The model under review builds one solid part; all positions refer to its coordinate system, in mm. A direction names the side the tool comes from. Coordinates: 2 decimals unless noted, no trailing zeros. Write each loop counter-clockwise with the first axis right and the second up, starting at its lowest first coordinate (ties: lowest second). Pieces come first, ordered by that corner, then holes. Notation, with made-up numbers: (-6, 36.5) - (38, 36.5) arc R9 cw to (38, 42.5) - close; hole circle Ø3 at (2.25, -27). An arc over 180 degrees is marked (long way). Put each result on its own line as item: value. Start each with the question number.
Item 1: Machinability: for faces 1 (the face through (1.115, 41.855, 5.022)), 2 (the face through (0.07, 13, 14.15)), 3 (the face through (-12.932, 6.409, 5.362)), which of the approach directions +Z, -Z, +X, -X, +Y, -Y give a long, thin tool a straight path to every point of the face, cutting with its end or side? Answer none if there is none.
Item 2: Consider section D-D on y = 40.5. Give the boundary of the cut face in (x, z), then the cut area to 3 significant figures.
Item 3: Consider section A-A on y = 5. State how many separate pieces and enclosed holes the cut face has, then the cut area to 3 significant figures.
Item 4: To check wall thickness, follow L1, parallel to Y at x = -11, z = -11; L2, parallel to Y at x = -10, z = -11; L3, parallel to X at y = 23.5, z = 1. State the ranges of each line that lie inside material, in increasing order. Write a range as [from, to].
Item 5: Consider section B-B on y = 23. Give the boundary of the cut face in (x, z).
Item 6: Mouldability with a two-part tool opening along X and no side actions: class faces 4 (the face through (4.119, 19.126, 18.548)), 5 (the face through (-6, 0, -13)), 6 (the face through (3.47, 19.78, 15.62)) as pulls with the +X half, pulls with the -X half, needs draft (parallel to the pull), parting line crosses it, or undercut.
Item 7: For pin 1 (10 mm diameter, centred on x = -6, z = -6.5, fed in from -Y); pin 2 (2 mm diameter, centred on y = 40.5, z = 8.5, fed in from -X); pin 3 (3 mm diameter, centred on x = 3, z = 2, fed in from -Y); pin 4 (1 mm diameter, centred on x = -10, y = 14.5, fed in from -Z), all flat-tipped, find the tip position at first contact; note any pin that passes through.
```python
from build123d import *

# Parameters (mm, degrees)
SKETCH3_R          = 1.5
CUT_EXTRUDE1_DEPTH = 55.138710735
CIRPATTERN1_COUNT  = 8


with BuildPart() as part:
    # Sketch2 → Revolve1 (revolve)
    with BuildSketch(Plane.XY, mode=Mode.PRIVATE) as revolve1_sk:
        Polygon((17, 0), (17, 10), (19, 10), (19, 28), (0, 47), (0, 42.757359313), (16, 26.757359313), (16, 13), (14, 13), (14, 0), align=None)
    revolve(revolve1_sk.sketch.rotate(Axis((0, 26.112729166, 0), (0, -1, 0)), 180), axis=Axis((0, 26.112729166, 0), (0, -1, 0)))

    # Sketch3 → Cut-Extrude1 (cut, through all)
    with BuildSketch(Plane.XY):
        with Locations((0, 5)):
            Circle(SKETCH3_R)
    cut_extrude1 = extrude(amount=-CUT_EXTRUDE1_DEPTH, mode=Mode.SUBTRACT)

    # CirPattern1: Cut-Extrude1 ×8 about axis
    cirpattern1_axis = Axis((0, 26.112729166, 0), (0, 1, 0))
    for i in range(1, CIRPATTERN1_COUNT):
        add(cut_extrude1.rotate(cirpattern1_axis, i * 360 / CIRPATTERN1_COUNT), mode=Mode.SUBTRACT)


solid = part.part
```
Report:
1. face 1: +Y
1. face 2: none
1. face 3: -Y
2. outline: circle Ø13 at (0, 0); hole circle Ø4.51 at (0, 0)
2. area: 117 mm²
3. separate pieces: 8
3. enclosed holes: 0
3. area: 220 mm²
4. L1: [0, 3.5], [6.5, 13], [27.2, 31.44]
4. L2: [0, 3.68], [6.32, 13], [27.89, 32.13]
4. L3: [-18.97, -15.97], [15.97, 18.97]
5. outline: circle Ø38 at (0, 0); hole circle Ø32 at (0, 0)
6. face 4: parting line crosses it
6. face 5: needs draft
6. face 6: undercut
7. pin 1: y = 28.91
7. pin 2: through
7. pin 3: y = 37.65
7. pin 4: z = -16.45
